```python
from build123d import *

# Parameters (mm, degrees)
BOSS_EXTRUDE1_DEPTH = 533.4
SKETCH2_R           = 5.715
CUT_EXTRUDE1_DEPTH  = 32.75


with BuildPart() as part:
    # Sketch1 → Boss-Extrude1 (new body, symmetric)
    with BuildSketch(Plane(origin=(0, 0, 0), x_dir=(1, 0, 0), z_dir=(0, 1, 0))):
        with BuildLine():
            Line((-9.525, -15.875), (9.525, -15.875))
            ThreePointArc((9.525, -15.875), (14.015128061, -14.015128061), (15.875, -9.525))
            Line((15.875, -9.525), (15.875, 9.525))
            ThreePointArc((15.875, 9.525), (14.015128061, 14.015128061), (9.525, 15.875))
            Line((9.525, 15.875), (-9.525, 15.875))
            ThreePointArc((-9.525, 15.875), (-14.015128061, 14.015128061), (-15.875, 9.525))
            Line((-15.875, 9.525), (-15.875, -9.525))
            ThreePointArc((-15.875, -9.525), (-14.015128061, -14.015128061), (-9.525, -15.875))
        make_face()
        with BuildLine():
            Line((-8.6995, -13.462), (8.6995, -13.462))
            ThreePointArc((8.6995, -13.462), (12.067096045, -12.067096045), (13.462, -8.6995))
            Line((13.462, -8.6995), (13.462, 8.0645))
            ThreePointArc((13.462, 8.0645), (12.067096045, 11.432096045), (8.6995, 12.827))
            Line((8.6995, 12.827), (-8.6995, 12.827))
            ThreePointArc((-8.6995, 12.827), (-12.067096045, 11.432096045), (-13.462, 8.0645))
            Line((-13.462, 8.0645), (-13.462, -8.6995))
            ThreePointArc((-13.462, -8.6995), (-12.067096045, -12.067096045), (-8.6995, -13.462))
        make_face(mode=Mode.SUBTRACT)
    extrude(amount=BOSS_EXTRUDE1_DEPTH, both=True)

    # Sketch2 → Cut-Extrude1 (cut, through all)
    with BuildSketch(Plane.XY.offset(15.875)):
        with Locations((0, 517.525)):
            Circle(SKETCH2_R)
    cut_extrude1 = extrude(amount=-CUT_EXTRUDE1_DEPTH, mode=Mode.SUBTRACT)

    # Mirror1: Cut-Extrude1 across plane
    add(cut_extrude1.mirror(Plane.ZX), mode=Mode.SUBTRACT)


solid = part.part
```
Geometry check sheet. Reference: the model listing, model coordinates, mm. A direction names the side the tool comes from. Give positions to 0.01 mm unless a question says otherwise; leave off trailing zeros. Loops run counter-clockwise (first coordinate to the right, second up) from the corner with the lowest first, then second, coordinate; pieces in that order, holes last. Notation, with made-up numbers: M 82,-24.5 L 86,-24.5 A21 ccw 86,-9.5 Z; hole C 30.25,18.25 d3. An arc over 180 degrees is marked long. Answer as CSV lines item,"result".
Item 1: Cross-section at A-A on x = 0. Record the cut outline in (y, z) (3 decimals).
Values:
outline,"M -533.4,-15.875 L -523.24,-15.875 L -523.24,-12.827 L -533.4,-12.827 Z; M -533.4,13.462 L -523.24,13.462 L -523.24,15.875 L -533.4,15.875 Z; M -511.81,-15.875 L 511.81,-15.875 L 511.81,-12.827 L -511.81,-12.827 Z; M -511.81,13.462 L 511.81,13.462 L 511.81,15.875 L -511.81,15.875 Z; M 523.24,-15.875 L 533.4,-15.875 L 533.4,-12.827 L 523.24,-12.827 Z; M 523.24,13.462 L 533.4,13.462 L 533.4,15.875 L 523.24,15.875 Z"
Item 2: Access from +Z, -Z, +X, -X, +Y, -Y to the whole of each face (thin tool, end or side, straight path). Record for faces 4 (the flat face through (0, 7, -12.827)), 5 (the flat face through (15.875, 7, 0)).
Values:
face 4,"+Y, -Y"
face 5,"+Z, -Z, +X, +Y, -Y"
Item 3: Cross-section at B-B on z = -0.5. Record the cut outline in (x, y) (3 decimals).
Values:
outline,"M -15.875,-533.4 L -13.462,-533.4 L -13.462,533.4 L -15.875,533.4 Z; M 13.462,-533.4 L 15.875,-533.4 L 15.875,533.4 L 13.462,533.4 Z"
Item 4: Material ranges on line 1 (Y direction, x = 0, z = -14); line 2 (Z direction, x = -9.5, y = 372.5) (3 decimals); line 3 (X direction, y = -18, z = 7.5) (3 decimals), recorded low to high.
Values:
line 1,"y = -533.4 to -523.24, -511.81 to 511.81, 523.24 to 533.4"
line 2,"z = -15.875 to -12.759, 13.394 to 15.875"
line 3,"x = -15.875 to -13.462, 13.462 to 15.875"
Item 5: Release check for a two-part mould opening along Z. For faces 1 (the flat face through (1, -533.4, -13)), 2 (the flat face through (0, 7, -15.875)), 3 (the flat face through (-13.462, 7, 0)) record: pulls with the +Z half, pulls with the -Z half, needs draft (parallel to the pull), parting line crosses it, or undercut.
Values:
face 1,"needs draft"
face 2,"pulls with the -Z half"
face 3,"undercut"
Item 6: Depth check by flat-ended pin: P1, Ø12, axis at y = -354.5, z = -10, coming from the -X side (3 decimals). Enter the tip coordinate at first touch or a pass-through.
Values:
P1,"stops at x = -15.875"
